CAD build for the part. Positions are in the model's coordinates, mm. Face numbers are marked on the shaded views. A direction names the side the tool comes from. Give positions to 0.01 mm unless a question says otherwise; leave off trailing zeros. Order: outer loops, then holes, each group sorted by start corner. A loop starts at its lowest first (then second) coordinate and runs counter-clockwise, first axis right, second up. Notation, with made-up numbers: (56, 32.25) -> (94, 32.25) arc R13 cw to (94, 36.25) -> close; hole circle Ø6 at (79.25, 71). An arc over 180 degrees is marked (long way). Answer as CSV lines item,"result".
```python
from build123d import *

# Parameters (mm, degrees)
F1_W     = 23.7
F1_H     = 36.5
F2_DEPTH = 9
F3_DEPTH = 7.5


with BuildPart() as f2:
    # F1 (on Top) → F2 (new body)
    with BuildSketch(Plane.XY):
        with Locations((0, 0.75)):
            Rectangle(F1_W, F1_H)
    extrude(amount=F2_DEPTH)

    # F0 (on Top) → F3 (cut)
    with BuildSketch(Plane.XY):
        Polygon((-10.35, -17.5), (10.35, -17.5), (10.35, 17.5), (2.75, 17.5), (2.75, 19), (-2.75, 19), (-2.75, 17.5), (-10.35, 17.5), align=None)
    extrude(amount=F3_DEPTH, mode=Mode.SUBTRACT)


solid = f2.part
```
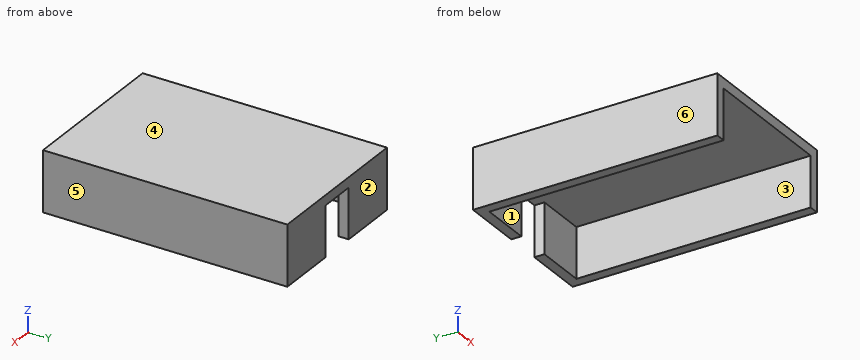
1) Which spindle directions (+Z, -Z, +X, -X, +Y, -Y) get a long thin tool onto all of the face, cutting with end or side? Do the marked faces 1 and 2. Say none if no direction does.
Data:
face 1,"-Z, -Y"
face 2,"+Z, -Z, +X, -X, +Y"
2) Band-saw the part on B-B, the plane y = 1. Write the cut outline in (x, z).
Data:
outline,"(-11.85, 0) -> (-10.35, 0) -> (-10.35, 7.5) -> (10.35, 7.5) -> (10.35, 0) -> (11.85, 0) -> (11.85, 9) -> (-11.85, 9) -> close"
3) Pin check, flat tips, straight feed: P1, Ø3, axis at x = -8, y = 15, coming from the -Z side; P2, Ø4, axis at x = -7, z = 3.5, coming from the -Y side. Stop position of each tip, or through.
Data:
P1,"stops at z = 7.5"
P2,"stops at y = 17.5"
4) Pull direction X, two halves, no side cores. Call the marked faces 3, 4, 5 and 6: pulls with the +X half, pulls with the -X half, needs draft (parallel to the pull), parting line crosses it, or undercut.
Data:
face 3,"undercut"
face 4,"needs draft"
face 5,"pulls with the +X half"
face 6,"pulls with the -X half"
5) Band-saw the part on A-A, the plane z = 6.75. Write the cut outline in (x, y).
Data:
outline,"(-11.85, -17.5) -> (-10.35, -17.5) -> (-10.35, 17.5) -> (-2.75, 17.5) -> (-2.75, 19) -> (-11.85, 19) -> close; (2.75, 17.5) -> (10.35, 17.5) -> (10.35, -17.5) -> (11.85, -17.5) -> (11.85, 19) -> (2.75, 19) -> close"
6) Band-saw the part on C-C, the plane x = -5. Write the cut outline in (y, z).
Data:
outline,"(-17.5, 7.5) -> (17.5, 7.5) -> (17.5, 0) -> (19, 0) -> (19, 9) -> (-17.5, 9) -> close"
7) Wall check: line 1 along X through (y, z) = (2, 5.25); line 2 along Y through (x, z) = (7.75, 2.5); line 3 along Z through (x, y) = (2.5, -11). Give the ranges that are in metal, low to high. Write a range as [from, to].
Data:
line 1,"x = [-11.85, -10.35], [10.35, 11.85]"
line 2,"y = [17.5, 19]"
line 3,"z = [7.5, 9]"
